Study the drawing (mm; zero at the part's minimum x, y, z) and answer. A direction names the side the tool comes from. Give positions to 0.01 mm unless a question says otherwise; leave off trailing zeros. Order: outer loops, then holes, each group sorted by start corner. A loop starts at its lowest first (then second) coordinate and runs counter-clockwise, first axis right, second up.
Item 1: A cutting plane is placed at A-A (z = 65). Write down the section's boundary in (x, y), plus the area to 3 significant figures.
Item 2: Find the intervals of material crossed by line 1 along Z through (x, y) = (39, 4.5); line 2 along X through (y, z) = (18, 108.25); line 3 along Z through (x, y) = (47, 17.5) (1 decimal), in increasing order.
Item 3: A cutting plane is placed at B-B (x = 90). Write down the section's boundary in (y, z).
Item 4: Which of the six approach directions +Z, -Z, +X, -X, +Y, -Y give full straight-line access (tool end or side, diameter ignored) to the marked faces 1 and 2?
Item 5: A cutting plane is placed at C-C (z = 108.25). Write down the section's boundary in (x, y).
Item 6: A cutting plane is placed at D-D (y = 11.5). Write down the section's boundary in (x, z), plus the area to 3 significant figures.
Item 7: Given pin 1 Ø4 at (x, z) = (11.43, 59.11) entering from -Y; pin 2 Ø5.5 at (x, z) = (48.25, 101.75) entering from -Y; pin 3 Ø11 at (y, z) = (16, 102.5) entering from +X; pin 4 Ø8 at (x, y) = (84, 7) entering from +Z, each flat-ended and moving along its own axis, determine where each tip first touches the part or whether it passes through.
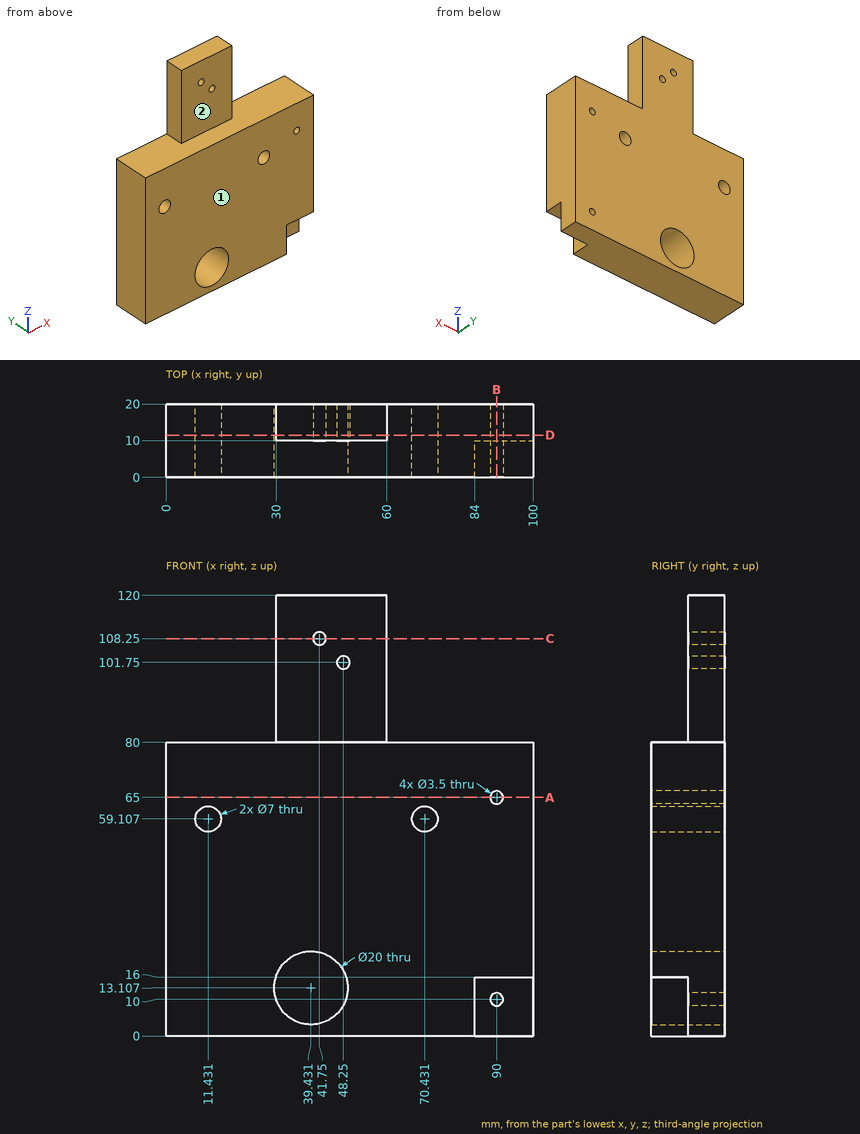
Response values:
1. outline: (0, 0) - (88.25, 0) - (88.25, 20) - (0, 20) - close; (91.75, 0) - (100, 0) - (100, 20) - (91.75, 20) - close
1. area: 1,930 mm2
2. line 1: z = 0 to 3.12, 23.1 to 80
2. line 2: x = 30 to 40, 43.5 to 60
2. line 3: z = 0 to 6.6, 19.6 to 100.5, 103 to 120
3. outline: (0, 16) - (10, 16) - (10, 11.75) - (20, 11.75) - (20, 63.25) - (0, 63.25) - close; (0, 66.75) - (20, 66.75) - (20, 80) - (0, 80) - close; (10, 0) - (20, 0) - (20, 8.25) - (10, 8.25) - close
4. face 1: +Z, -Z, +X, -X, -Y
4. face 2: +Z, +X, -X, -Y
5. outline: (30, 10) - (40, 10) - (40, 20) - (30, 20) - close; (43.5, 10) - (60, 10) - (60, 20) - (43.5, 20) - close
6. outline: (0, 0) - (100, 0) - (100, 80) - (60, 80) - (60, 120) - (30, 120) - (30, 80) - (0, 80) - close; hole circle Ø7 at (11.43, 59.11); hole circle Ø20 at (39.43, 13.11); hole circle Ø3.5 at (41.75, 108.25); hole circle Ø3.5 at (48.25, 101.75); hole circle Ø7 at (70.43, 59.11); hole circle Ø3.5 at (90, 10); hole circle Ø3.5 at (90, 65)
6. area: 8,770 mm2
7. pin 1: passes through
7. pin 2: stops at y = 10
7. pin 3: stops at x = 60
7. pin 4: stops at z = 80
